```python
from build123d import *


with BuildPart() as part:
    # Sketch1 → Revolve1 (revolve)
    with BuildSketch(Plane.XY):
        with BuildLine():
            Line((0, 0), (2.38, 0))
            Line((2.38, 0), (2.38, 6.35))
            Line((2.38, 6.35), (4.77, 6.35))
            Line((4.77, 6.35), (4.77, 6.635226112))
            ThreePointArc((4.77, 6.635226112), (5.668747391, 10.685686779), (9.4, 12.5))
            ThreePointArc((9.4, 12.5), (15.237749216, 16.587689011), (10.5, 21.911432968))
            Line((10.5, 21.911432968), (0, 21.911432968))
            Line((0, 21.911432968), (0, 0))
        make_face()
    revolve(axis=Axis((0, 0, 0), (0, 1, 0)))


solid = part.part
```
Build history of the part. All positions in model axes, mm. A direction names the side the tool comes from. Give positions to 0.01 mm unless a question says otherwise; leave off trailing zeros. Order: outer loops, then holes, each group sorted by start corner. A loop starts at its lowest first (then second) coordinate and runs counter-clockwise, first axis right, second up. Notation, with made-up numbers: M -26,22 L 20,22 A23 cw 20,52 Z; hole C 35,14 d4. An arc over 180 degrees is marked long. Write item = value, one per line. Start each with the question number.
(1) Slice it at B-B on x = 0. Write the cut outline in (y, z), plus the area to 3 significant figures.
(2) Slice it at C-C on y = 4.25. Write the cut outline in (x, z), plus the area to 3 significant figures.
(3) Probe L1, parallel to Z at x = 7.5, y = 13.5; L2, parallel to Y at x = 2.5, z = -0.5; L3, parallel to Z at x = 3.5, y = 9.5. List the from-to ranges inside material, lowest first. Write a range as [from, to].
(4) Slice it at A-A on z = 0. Write the cut outline in (x, y).
(5) Which spindle directions (+Z, -Z, +X, -X, +Y, -Y) get a long thin tool onto all of the face, cutting with end or side? Do faces 1 (the flat face through (0, 0, 0)), 2 (the cylindrical face through (-0.516, 3.219, 2.323)). Say none if no direction does.
(6) Pin check, flat tips, straight feed: pin 1 Ø2 at (y, z) = (9, -7) entering from -X; pin 2 Ø2 at (y, z) = (14, -8) entering from -X; pin 3 Ø1 at (x, z) = (-6, -6.5) entering from -Y; pin 4 Ø1 at (y, z) = (14.5, 7) entering from +X. Stop position of each tip, or through.
(7) Slice it at D-D on y = 10.25. Write the cut outline in (x, z).
Responses:
q1.outline = M 0,-2.38 L 6.35,-2.38 L 6.35,-4.77 L 6.64,-4.77 A4.77 cw 12.5,-9.4 A4.77 ccw long 21.91,-10.5 L 21.91,10.5 A4.77 ccw long 12.5,9.4 A4.77 cw 6.64,4.77 L 6.35,4.77 L 6.35,2.38 L 0,2.38 Z
q1.area = 367 mm2
q2.outline = C 0,0 d4.76
q2.area = 17.8 mm2
q3.L1 = [-11.32, 11.32]
q3.L2 = [6.35, 21.91]
q3.L3 = [-3.55, 3.55]
q4.outline = M -10.5,21.91 A4.77 ccw long -9.4,12.5 A4.77 cw -4.77,6.64 L -4.77,6.35 L -2.38,6.35 L -2.38,0 L 2.38,0 L 2.38,6.35 L 4.77,6.35 L 4.77,6.64 A4.77 cw 9.4,12.5 A4.77 ccw long 10.5,21.91 Z
q5.face_1 = +Z, -Z, +X, -X, -Y
q5.face_2 = -Y
q6.pin_1 = through
q6.pin_2 = -12.65
q6.pin_3 = 12.38
q6.pin_4 = 13.1
q7.outline = C 0,0 d10.73
